```python
from build123d import *

# Parameters (mm, degrees)
SKETCH2_R           = 20
SKETCH2_R_2         = 17.5
BOSS_EXTRUDE1_DEPTH = 30
SKETCH3_R           = 20
SKETCH3_R_2         = 17.5
BOSS_EXTRUDE2_DEPTH = 30
BOSS_EXTRUDE3_DEPTH = 5
SKETCH5_R           = 13
SKETCH5_R_2         = 10
BOSS_EXTRUDE4_DEPTH = 30


with BuildPart() as part:
    # Sketch2 → Boss-Extrude1 (new body)
    with BuildSketch(Plane.XY.offset(-35.355)):
        Circle(SKETCH2_R)
        Circle(SKETCH2_R_2, mode=Mode.SUBTRACT)
    extrude(amount=-BOSS_EXTRUDE1_DEPTH)



with BuildPart() as body_2:
    # Sketch3 → Boss-Extrude2 (new body)
    with BuildSketch(Plane.XY.offset(35.355)):
        Circle(SKETCH3_R)
        Circle(SKETCH3_R_2, mode=Mode.SUBTRACT)
    extrude(amount=BOSS_EXTRUDE2_DEPTH)


with BuildPart() as part_1:
    add(part.part)

    add(body_2.part)  # Boss-Extrude3 merges body 2
    # Sketch4 → Boss-Extrude3 (add, symmetric)
    with BuildSketch(Plane(origin=(0, 0, 0), x_dir=(1, 0, 0), z_dir=(0, 1, 0))):
        Polygon((18.5, -65.355), (18.5, -35.355), (518.5, -35.355), (553.5, -12.138626468), (553.5, 12.138626468), (518.5, 35.355), (18.5, 35.355), (18.5, 65.355), (518.5, 65.355), (578.5, 25.555502516), (578.5, -25.555502516), (518.5, -65.355), align=None)
    extrude(amount=BOSS_EXTRUDE3_DEPTH, both=True)

    # Sketch5 → Boss-Extrude4 (add, symmetric)
    with BuildSketch(Plane.XY):
        with Locations((589, 0)):
            Circle(SKETCH5_R)
        with Locations((589, 0)):
            Circle(SKETCH5_R_2, mode=Mode.SUBTRACT)
    extrude(amount=BOSS_EXTRUDE4_DEPTH, both=True)


solid = part_1.part
```
Work out the finished part from the listing and answer in its coordinate system (mm). A direction names the side the tool comes from. Give positions to 0.01 mm unless a question says otherwise; leave off trailing zeros. Loops run counter-clockwise (first coordinate to the right, second up) from the corner with the lowest first, then second, coordinate; pieces in that order, holes last. Notation, with made-up numbers: (79.5, 1.5) - (115.5, 1.5) arc R34 ccw to (115.5, 35.5) - close; hole circle Ø11 at (37.5, 46). An arc over 180 degrees is marked (long way). Use CSV: the item, a comma, the result in double quotes. Start each with the question number.
(1) Find section A-A, the plane x = 91. Determine the outline of the cut face in (y, z) (3 decimals).
(2) Find section D-D, the plane x = 589. Determine the outline of the cut face in (y, z).
(3) Find section C-C, the plane z = 47. Determine the outline of the cut face in (x, y), plus the area to 3 significant figures.
(4) Each of these flat-tipped pins is pushed along its axis until it touches: pin 1 (10 mm diameter, centred on x = 105.5, z = 49.5, fed in from -Y); pin 2 (1 mm diameter, centred on x = 469, y = 6, fed in from +Z); pin 3 (1 mm diameter, centred on y = 4, z = 25, fed in from +X); pin 4 (1.5 mm diameter, centred on y = 2, z = -38, fed in from -X). Where does it stop, or does it pass through?
(5) Find the intervals of material crossed by L1, parallel to Y at x = 0, z = 50; L2, parallel to Z at x = 20.5, y = 2 (3 decimals); L3, parallel to Y at x = 589, z = 7.5, in increasing order.
(6) Find section B-B, the plane x = 0. Determine the outline of the cut face in (y, z) (3 decimals).
(7) A tool of negligible diameter and unlimited length cuts with its end or side. For faces 1 (the face through (596, -8, -30)), 2 (the face through (535.755, 0.07, 23.909)), 3 (the face through (-19.984, 0.809, -50.145)), from which of +Z, -Z, +X, -X, +Y, -Y can it reach the whole face along a straight path? Write none if from no direction.
(8) Determine the mould class of faces 4 (the face through (-19.984, 0.809, 50.145)), 5 (the face through (596, -8, 30)), 6 (the face through (-13.887, -10.648, 50.145)) for opening direction Y: released by +Y, released by -Y, zero draft, split by the parting line, or undercut.
Results found:
1,outline,"(-5, -65.355) - (5, -65.355) - (5, -35.355) - (-5, -35.355) - close; (-5, 35.355) - (5, 35.355) - (5, 65.355) - (-5, 65.355) - close"
2,outline,"(-13, -30) - (-10, -30) - (-10, 30) - (-13, 30) - close; (10, -30) - (13, -30) - (13, 30) - (10, 30) - close"
3,outline,"(19.36, -5) - (546.17, -5) - (546.17, 5) - (19.36, 5) arc R20 ccw (long way) to start; hole circle Ø35 at (0, 0)"
3,area,"5,560 mm^2"
4,pin 1,"y = -5"
4,pin 2,"through"
4,pin 3,"x = 601.52"
4,pin 4,"x = -19.96"
5,L1,"-20 to -17.5, 17.5 to 20"
5,L2,"-65.355 to -35.355, 35.355 to 65.355"
5,L3,"-13 to -10, 10 to 13"
6,outline,"(-20, -65.355) - (-17.5, -65.355) - (-17.5, -35.355) - (-20, -35.355) - close; (-20, 35.355) - (-17.5, 35.355) - (-17.5, 65.355) - (-20, 65.355) - close; (17.5, -65.355) - (20, -65.355) - (20, -35.355) - (17.5, -35.355) - close; (17.5, 35.355) - (20, 35.355) - (20, 65.355) - (17.5, 65.355) - close"
7,face 1,"-Z, +X, +Y, -Y"
7,face 2,"-X, +Y, -Y"
7,face 3,"+Z, -Z"
8,face 4,"split by the parting line"
8,face 5,"zero draft"
8,face 6,"undercut"
